The listing builds one solid part. Answer for the finished solid, in the listing's coordinates (mm). A direction names the side the tool comes from. Give positions to 0.01 mm unless a question says otherwise; leave off trailing zeros. Loops run counter-clockwise (first coordinate to the right, second up) from the corner with the lowest first, then second, coordinate; pieces in that order, holes last. Notation, with made-up numbers: (-19.75, -18.5) - (-6.75, -18.5) arc R23 cw to (-6.75, 5.5) - close; hole circle Ø10 at (-22, 72). An arc over 180 degrees is marked (long way). Answer in a Markdown table with one row per item. Add a question column.
```python
from build123d import *

# Parameters (mm, degrees)
F0_R     = 3
F1_DEPTH = 6
F3_R     = 1
F5_DEPTH = 18


with BuildPart() as f1:
    # F0 (on Top) → F1 (new body)
    with BuildSketch(Plane.XY):
        with BuildLine():
            Line((-15, -14), (15, -14))
            Line((15, -14), (15, 0))
            ThreePointArc((15, 0), (10.8994949366, 9.8994949366), (1, 14))
            Line((1, 14), (-1, 14))
            ThreePointArc((-1, 14), (-10.8994949366, 9.8994949366), (-15, 0))
            Line((-15, 0), (-15, -14))
        make_face()
        with Locations((0, 9.1889705509)):
            Circle(F0_R, mode=Mode.SUBTRACT)
    extrude(amount=F1_DEPTH)

    # F3
    f3_edges = [f1.edges().sort_by_distance(p)[0] for p in [
        (-10.899495, 9.899495, 6),
        (10.899495, 9.899495, 6),
        (-15, -7, 6),
        (15, -7, 6),
        (-15, -7, 0),
        (-10.899495, 9.899495, 0),
        (10.899495, 9.899495, 0),
        (15, -7, 0),
    ]]
    fillet(f3_edges, radius=F3_R)

    # F4 (on face) → F5 (join)
    with BuildSketch(Plane.XZ.offset(14)):
        with BuildLine():
            Line((-10.1717880173, 6), (-14, 0))
            Line((-14, 0), (-12.8137921418, 0))
            Line((-12.8137921418, 0), (-9.5468121047, 5.120374815))
            Line((-9.5468121047, 5.120374815), (-6.3790735405, 0))
            Line((-6.3790735405, 0), (-5.122384561, 0))
            Line((-5.122384561, 0), (-1.8554045239, 5.120374815))
            Line((-1.8554045239, 5.120374815), (1.3123340403, 0))
            Line((1.3123340403, 0), (2.5690230199, 0))
            Line((2.5690230199, 0), (5.836003057, 5.120374815))
            Line((5.836003057, 5.120374815), (9.0037416211, 0))
            Line((9.0037416211, 0), (10.2604306007, 0))
            Line((10.2604306007, 0), (14.0862641777, 5.9962722979))
            ThreePointArc((14.0862641777, 5.9962722979), (14.043172341, 5.9990676398), (14, 6))
            Line((14, 6), (12.9024347251, 6))
            Line((12.9024347251, 6), (9.635454688, 0.879625185))
            Line((9.635454688, 0.879625185), (6.4677161239, 6))
            Line((6.4677161239, 6), (5.2110271443, 6))
            Line((5.2110271443, 6), (1.9440471072, 0.879625185))
            Line((1.9440471072, 0.879625185), (-1.223691457, 6))
            Line((-1.223691457, 6), (-2.4803804365, 6))
            Line((-2.4803804365, 6), (-5.7473604736, 0.879625185))
            Line((-5.7473604736, 0.879625185), (-8.9150990378, 6))
            Line((-8.9150990378, 6), (-10.1717880173, 6))
        make_face()
    extrude(amount=F5_DEPTH)


solid = f1.part
```
(1) A cutting plane is placed at B-B on y = -21. Determine the outline of the cut face in (x, z), plus the area to 3 significant figures.
(2) The mould has two halves that part along X. Classify faces 1 (the face through (0, -32, 3)), 2 (the face through (-12.06, -22.87, 3.04)), 3 (the face through (6, -14, 2)): pulls with the +X half, pulls with the -X half, needs draft (parallel to the pull), parting line crosses it, or undercut.
(3) Find the intervals of material crossed by line 1 along Y through (x, z) = (0, 3.35); line 2 along X through (y, z) = (0.5, 3.25); line 3 along X through (y, z) = (7.5, 1.5), in increasing order. Write a range as [from, to].
(4) A tool of negligible diameter and unlimited length cuts with its end or side. For faces 4 (the face through (4.18, -22.874, 2.524)), 5 (the face through (8.074, -22.874, 3.404)), 6 (the face through (12.15, -22.87, 2.96)), from which of +Z, -Z, +X, -X, +Y, -Y can it reach the whole face along a straight path? Write none if from no direction.
(5) Given pin 1 Ø1 at (x, z) = (2, 1) entering from +Y, flat-ended and moving along its own axis, determine where the tip first touches the part or whether it passes through.
(6) A cutting plane is placed at A-A on x = 0. Determine the outline of the cut face in (y, z).
Evaluation:
| question | item | result |
|---|---|---|
| 1 | outline | (-14, 0) - (-12.81, 0) - (-9.55, 5.12) - (-6.38, 0) - (-5.12, 0) - (-1.86, 5.12) - (1.31, 0) - (2.57, 0) - (5.84, 5.12) - (9, 0) - (10.26, 0) - (14.09, 6) arc R1 ccw to (14, 6) - (12.9, 6) - (9.64, 0.88) - (6.47, 6) - (5.21, 6) - (1.94, 0.88) - (-1.22, 6) - (-2.48, 6) - (-5.75, 0.88) - (-8.92, 6) - (-10.17, 6) - close |
| 1 | area | 46.7 mm² |
| 2 | face 1 | needs draft |
| 2 | face 2 | pulls with the -X half |
| 2 | face 3 | undercut |
| 3 | line 1 | y = [-32, 6.19], [12.19, 14] |
| 3 | line 2 | x = [-14.99, 14.99] |
| 3 | line 3 | x = [-12.82, -2.48], [2.48, 12.82] |
| 4 | face 4 | -Z, -Y |
| 4 | face 5 | +Z, -Y |
| 4 | face 6 | -Z, +X, -Y |
| 5 | pin 1 | stops at y = 13.99 |
| 6 | outline | (-32, 2.12) - (-14, 2.12) - (-14, 0) - (6.19, 0) - (6.19, 6) - (-14, 6) - (-14, 4.02) - (-32, 4.02) - close; (12.19, 0) - (13, 0) arc R1 ccw to (14, 1) - (14, 5) arc R1 ccw to (13, 6) - (12.19, 6) - close |
